from build123d import *

# Parameters (mm, degrees)
REDONDEO2_R           = 10
CROQUIS3_R            = 14.85
CORTAR_EXTRUIR1_DEPTH = 10
CROQUIS4_R            = 3.35
CROQUIS4_R_2          = 4
CROQUIS4_R_3          = 4.1
CROQUIS4_R_4          = 4.05
CORTAR_EXTRUIR2_DEPTH = 10
REDONDEO3_R           = 10
REDONDEO4_R           = 1


with BuildPart() as part:
    # Croquis2 → Revolución1 (revolve)
    with BuildSketch(Plane.XY, mode=Mode.PRIVATE) as revoluci_n1_sk:
        Polygon((54.45, 0), (71.45, 0), (71.45, 10), (69.45, 10), (69.45, 32.4), (71.45, 32.4), (71.45, 34.4), (38.5, 34.4), (38.5, 41.25), (0, 41.25), (0, 38.25), (35.5, 38.25), (35.5, 31.4), (54.45, 31.4), align=None)
    revolve(revoluci_n1_sk.sketch.rotate(Axis((0, 41.25, 0), (0, -1, 0)), 90), axis=Axis((0, 41.25, 0), (0, -1, 0)))

    # Redondeo2
    # the kernel refuses this fillet: 10 mm, written as the material it takes off along each edge
    with BuildSketch(Plane(origin=(0, 41.25, 0), x_dir=(0, 0, 1), z_dir=(1, 0, 0))) as redondeo2_piece_1:
        with BuildLine():
            CenterArc((29.00908329, 10), REDONDEO2_R, 270, 71.639186206)
            Line((29.00908329, 0), (29.00908329, -0.2))
            Line((29.00908329, -0.2), (38.5, -0.2))
            Line((38.5, -0.2), (38.7, 0))
            ThreePointArc((38.7, 0), (38.7, 3.425), (38.689818334, 6.787))
            Line((38.689818334, 6.787), (38.5, 6.85))
        make_face()
    revolve(axis=Axis((0, 41.25, 0), (0, -1, 0)), mode=Mode.SUBTRACT)

    # Croquis3 → Cortar-Extruir1 (cut)
    with BuildSketch(Plane(origin=(0, 41.25, 0), x_dir=(1, 0, 0), z_dir=(0, 1, 0))):
        with Locations(Location((0, 0, 0), (0, 0, 270))):
            Circle(CROQUIS3_R)
    extrude(amount=-CORTAR_EXTRUIR1_DEPTH, mode=Mode.SUBTRACT)

    # Croquis4 → Cortar-Extruir2 (cut)
    with BuildSketch(Plane(origin=(0, 41.25, 0), x_dir=(1, 0, 0), z_dir=(0, 1, 0))):
        with Locations(Location((0.518366506, 19.743196199, 0), (0, 0, 270))):
            Circle(CROQUIS4_R)
        with Locations(Location((-16.5, 10.854146673, 0), (0, 0, 270))):
            Circle(CROQUIS4_R_2)
        with Locations(Location((16.5, 10.854146673, 0), (0, 0, 270))):
            Circle(CROQUIS4_R_2)
        with Locations(Location((16.5, -10.854146673, 0), (0, 0, 270))):
            Circle(CROQUIS4_R_3)
        with Locations(Location((-16.5, -10.854146673, 0), (0, 0, 270))):
            Circle(CROQUIS4_R_4)
    extrude(amount=-CORTAR_EXTRUIR2_DEPTH, mode=Mode.SUBTRACT)

    # Redondeo3
    # the kernel refuses this fillet: 10 mm, written as the material it takes off along each edge
    with BuildSketch(Plane(origin=(0, 31.4, 0), x_dir=(0, 0, 1), z_dir=(1, 0, 0))) as redondeo3_piece_1:
        with BuildLine():
            CenterArc((44.99091671, -10), REDONDEO3_R, 90, 71.639186206)
            Line((35.5, -6.85), (35.310181666, -6.787))
            ThreePointArc((35.310181666, -6.787), (35.3, -3.425), (35.3, 0))
            Line((35.3, 0), (35.5, 0.2))
            Line((35.5, 0.2), (44.99091671, 0.2))
            Line((44.99091671, 0.2), (44.99091671, 0))
        make_face()
    revolve(axis=Axis((0, 31.4, 0), (0, -1, 0)), mode=Mode.SUBTRACT)

    # Redondeo4
    redondeo4_edges = [part.edges().sort_by_distance(p)[0] for p in [
        (0, 31.4, -54.45),
    ]]
    fillet(redondeo4_edges, radius=REDONDEO4_R)


solid = part.part
Geometry check sheet. Reference: the model listing, model coordinates, mm. A direction names the side the tool comes from. Round coordinates to 2 decimals unless told otherwise and drop trailing zeros. Order: outer loops, then holes, each group sorted by start corner. A loop starts at its lowest first (then second) coordinate and runs counter-clockwise, first axis right, second up. Notation, with made-up numbers: M 63.5,7 L 105.5,7 A9 ccw 105.5,16 Z; hole C -35.75,15 d10. An arc over 180 degrees is marked long. Answer in a Markdown table with one row per item.
(1) Tool access check on faces 5 (the face through (39, 31.4, 24)), 6 (the face through (-68.86, 21.36, -9.04)), 7 (the face through (-3.14, 33.41, -71.38)). Record the directions out of +Z, -Z, +X, -X, +Y, -Y that give a thin tool (end or side, any length) a straight path to the whole face; none if there is none.
Responses:
| item | result |
|---|---|
| face 5 | -Y |
| face 6 | none |
| face 7 | +Y, -Y |
(2) Draft check along Y on faces 1 (the face through (31, 34.4, 31)), 2 (the face through (-13.797, 39.771, -13.802)), 3 (the face through (15, 38.25, 0)), 4 (the face through (-59, 32.4, 37)). Enter one of: released by +Y, released by -Y, zero draft, split by the parting line, or undercut.
Responses:
| item | result |
|---|---|
| face 1 | released by +Y |
| face 2 | zero draft |
| face 3 | released by -Y |
| face 4 | undercut |
(3) Sectioned sample at C-C, the plane y = 4. Record the cut outline in (x, z).
Responses:
| item | result |
|---|---|
| outline | C 0,0 d142.9; hole C 0,0 d108.9 |
(4) Sectioned sample at B-B, the plane y = 26.5. Record the cut outline in (x, z), and give its area (3 significant figures).
Responses:
| item | result |
|---|---|
| outline | C 0,0 d138.9; hole C 0,0 d108.9 |
| area | 5,840 mm² |
(5) Scan lines: probe 1 along X at (y, z) = (39.5, 8); probe 2 along Z at (x, y) = (16, 39); probe 3 along X at (y, z) = (39.05, 0). Record each from-to range of solid material in increasing order. Write a range as from..to.
Responses:
| item | result |
|---|---|
| probe 1 | x = -33.72..-19.37, -13.63..-12.51, 12.51..13.56, 19.44..33.72 |
| probe 2 | z = -31.5..-14.82, -6.89..6.78, 14.92..31.5 |
| probe 3 | x = -35.27..-14.85, 14.85..35.27 |
(6) Go/stop test with flat-tipped pins: P1, Ø4, axis at x = 8.5, y = 26.5, coming from the +Z side; P2, Ø13, axis at x = -16.5, z = 10.85, coming from the +Y side; P3, Ø3, axis at x = -9.5, y = 30.5, coming from the +Z side; P4, Ø10, axis at y = 4, z = -35, coming from the +X side. Record where each tip stops, or that it passes through.
Responses:
| item | result |
|---|---|
| P1 | stops at z = 69.15 |
| P2 | stops at y = 41.25 |
| P3 | stops at z = 68.99 |
| P4 | stops at x = 64.85 |
